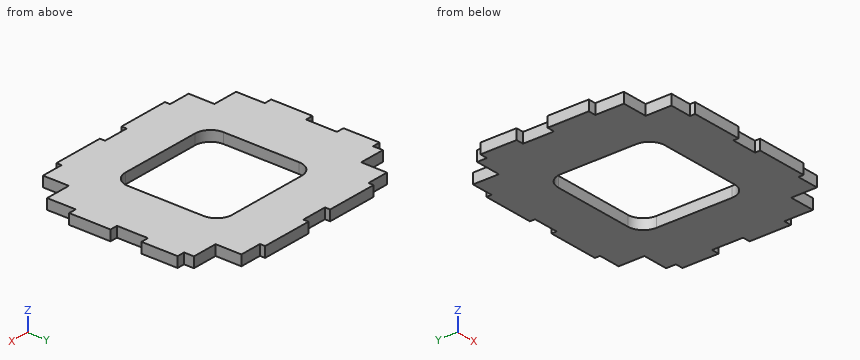
```python
from build123d import *

# Parameters (mm, degrees)
EXTRUDE_1_DEPTH = 2


with BuildPart() as part:
    # Model → 凸台-拉伸1 (new body)
    with BuildSketch(Plane.XY):
        Polygon((32.060999065, 47.930306361), (36.340999065, 47.930306361), (36.340999065, 48.930662067), (46.340999065, 48.930662067), (46.340999065, 47.930306361), (51.340999065, 47.930306361), (51.340999065, 48.930662067), (61.340999065, 48.930662067), (61.340999065, 47.930306361), (65.620999065, 47.930306361), (65.620999065, 42.930306361), (70.620999065, 42.930306361), (70.620999065, 41.030306361), (72.120999065, 41.030306361), (72.120999065, 34.030306361), (70.620999065, 34.030306361), (70.620999065, 28.030306361), (72.120999065, 28.030306361), (72.120999065, 20.030306361), (70.620999065, 20.030306361), (70.620999065, 14.488230775), (65.620999065, 14.488230775), (65.620999065, 9.488230775), (61.340999065, 9.488230775), (61.340999065, 8.487875069), (51.340999065, 8.487875069), (51.340999065, 9.488230775), (46.340999065, 9.488230775), (46.340999065, 8.487875069), (36.340999065, 8.487875069), (36.340999065, 9.488230775), (32.060999065, 9.488230775), (32.060999065, 14.488230775), (27.060999065, 14.488230775), (27.060999065, 20.030306361), (25.560999065, 20.030306361), (25.560999065, 28.030306361), (27.060999065, 28.030306361), (27.060999065, 34.030306361), (25.560999065, 34.030306361), (25.560999065, 41.030306361), (27.060999065, 41.030306361), (27.060999065, 42.930306361), (32.060999065, 42.930306361), align=None)
        with BuildLine():
            Line((56.992719614, 38.886063343), (40.972719614, 38.886063343))
            ThreePointArc((40.972719614, 38.886063343), (38.85139927, 38.007383686), (37.972719614, 35.886063343))
            Line((37.972719614, 35.886063343), (37.972719614, 21.236063342))
            ThreePointArc((37.972719614, 21.236063342), (38.85139927, 19.114742999), (40.972719614, 18.236063342))
            Line((40.972719614, 18.236063342), (56.992719614, 18.236063342))
            ThreePointArc((56.992719614, 18.236063342), (59.114039957, 19.114742999), (59.992719614, 21.236063342))
            Line((59.992719614, 21.236063342), (59.992719614, 35.886063343))
            ThreePointArc((59.992719614, 35.886063343), (59.114039957, 38.007383686), (56.992719614, 38.886063343))
        make_face(mode=Mode.SUBTRACT)
    extrude(amount=EXTRUDE_1_DEPTH)


solid = part.part
```
Work out the finished part from the listing and answer in its coordinate system (mm). Round coordinates to 2 decimals unless told otherwise and drop trailing zeros. Loops run counter-clockwise (first coordinate to the right, second up) from the corner with the lowest first, then second, coordinate; pieces in that order, holes last.
(1) The part is cut by section A-A, the plane x = 49. Give the vertices of the cut face in (y, z).
Computed values:
outline: (9.49, 0) - (18.24, 0) - (18.24, 2) - (9.49, 2) - close; (38.89, 0) - (47.93, 0) - (47.93, 2) - (38.89, 2) - close
(2) Each of these flat-tipped pins is pushed along its axis until it touches: P1, Ø1, axis at x = 28.5, z = 1.5, coming from the +Y side; P2, Ø0.8, axis at x = 26.5, z = 1, coming from the -Y side; P3, Ø0.8, axis at x = 71.5, z = 0.5, coming from the +Y side. Where does it stop, or does it pass through?
Computed values:
P1: stops at y = 42.93
P2: stops at y = 20.03
P3: stops at y = 41.03
(3) The part is cut by section D-D, the plane y = 11.5. Give the vertices of the cut face in (x, z).
Computed values:
outline: (32.06, 0) - (65.62, 0) - (65.62, 2) - (32.06, 2) - close
(4) Find the intervals of material crossed by L1, parallel to Y at x = 44, z = 1.95; L2, parallel to X at y = 26, z = 1.4; L3, parallel to Y at x = 47.5, z = 0.7, in increasing order.
Computed values:
L1: y = 8.49 to 18.24, 38.89 to 48.93
L2: x = 25.56 to 37.97, 59.99 to 72.12
L3: y = 9.49 to 18.24, 38.89 to 47.93
(5) The part is cut by section C-C, the plane x = 31. Give the vertices of the cut face in (y, z), and give its area (3 significant figures).
Computed values:
outline: (14.49, 0) - (42.93, 0) - (42.93, 2) - (14.49, 2) - close
area: 56.9 mm2
(6) The part is cut by section B-B, the plane y = 25. Give the vertices of the cut face in (x, z), and give its area (3 significant figures).
Computed values:
outline: (25.56, 0) - (37.97, 0) - (37.97, 2) - (25.56, 2) - close; (59.99, 0) - (72.12, 0) - (72.12, 2) - (59.99, 2) - close
area: 49.1 mm2
